Part model, mm, in its own coordinate system. Give positions to 0.01 mm unless a question says otherwise; leave off trailing zeros. Order: outer loops, then holes, each group sorted by start corner. A loop starts at its lowest first (then second) coordinate and runs counter-clockwise, first axis right, second up.
1. Slice it at A-A on z = -36.5. List the corners of the cut face in (x, y).
2. Slice it at B-B on y = -2.45. Give the number of separate pieces and of enclosed holes in the cut face, and give its area (3 significant figures).
3. Probe line 1 (X direction, y = -0.95, z = -402); line 2 (Z direction, x = 346, y = -0.75). List the from-to ranges inside material, lowest first.
from build123d import *

# Parameters (mm, degrees)
SKETCH1_W          = 434.8
SKETCH1_H          = 480.4
SKETCH1_W_2        = 2.7888
SKETCH1_H_2        = 220.2
BASE_FLANGE2_DEPTH = 3.264


# Sheet-metal steps are written as plain solids
with BuildPart() as part:
    # Sketch1 → Base-Flange2 (new body)
    with BuildSketch(Plane(origin=(0, 0, 0), x_dir=(1, 0, 0), z_dir=(0, 1, 0))):
        with Locations((217.4, 240.2)):
            Rectangle(SKETCH1_W, SKETCH1_H)
        with Locations((87.74, 355.8112)):
            Rectangle(SKETCH1_W_2, SKETCH1_H_2, mode=Mode.SUBTRACT)
        with Locations((87.74, 124.5888)):
            Rectangle(SKETCH1_W_2, SKETCH1_H_2, mode=Mode.SUBTRACT)
        with Locations((174.18, 355.8112)):
            Rectangle(SKETCH1_W_2, SKETCH1_H_2, mode=Mode.SUBTRACT)
        with Locations((174.18, 124.5888)):
            Rectangle(SKETCH1_W_2, SKETCH1_H_2, mode=Mode.SUBTRACT)
        with Locations((260.62, 355.8112)):
            Rectangle(SKETCH1_W_2, SKETCH1_H_2, mode=Mode.SUBTRACT)
        with Locations((260.62, 124.5888)):
            Rectangle(SKETCH1_W_2, SKETCH1_H_2, mode=Mode.SUBTRACT)
        with Locations((347.06, 355.8112)):
            Rectangle(SKETCH1_W_2, SKETCH1_H_2, mode=Mode.SUBTRACT)
        with Locations((347.06, 124.5888)):
            Rectangle(SKETCH1_W_2, SKETCH1_H_2, mode=Mode.SUBTRACT)
    extrude(amount=-BASE_FLANGE2_DEPTH)


solid = part.part
Data:
1. outline: (0, -3.26) - (86.35, -3.26) - (86.35, 0) - (0, 0) - close; (89.13, -3.26) - (172.79, -3.26) - (172.79, 0) - (89.13, 0) - close; (175.57, -3.26) - (259.23, -3.26) - (259.23, 0) - (175.57, 0) - close; (262.01, -3.26) - (345.67, -3.26) - (345.67, 0) - (262.01, 0) - close; (348.45, -3.26) - (434.8, -3.26) - (434.8, 0) - (348.45, 0) - close
2. separate pieces: 1
2. enclosed holes: 8
2. area: 204,000 mm2
3. line 1: x = 0 to 86.35, 89.13 to 172.79, 175.57 to 259.23, 262.01 to 345.67, 348.45 to 434.8
3. line 2: z = -480.4 to -465.91, -245.71 to -234.69, -14.49 to 0
